from build123d import *

# Parameters (mm, degrees)
EXTRUDE_1_DEPTH = 2
SKETCH_4_R      = 5.25
SKETCH_4_R_2    = 3.25
EXTRUDE_4_DEPTH = 42.99


with BuildPart() as part:
    # Эскиз1 → Бобышка-Вытянуть1 (new body)
    with BuildSketch(Plane(origin=(0, 0, 0), x_dir=(1, 0, 0), z_dir=(0, 1, 0))):
        with BuildLine():
            Line((-21.495, 0), (21.495, 0))
            Line((21.495, 0), (21.495, -55.974685573))
            ThreePointArc((21.495, -55.974685573), (11.495, -64.530824352), (17.994657773, -75.974685573))
            Line((17.994657773, -75.974685573), (12.58, -130))
            Line((12.58, -130), (-12.58, -130))
            Line((-12.58, -130), (-17.994657773, -75.974685573))
            ThreePointArc((-17.994657773, -75.974685573), (-11.495, -64.530824352), (-21.495, -55.974685573))
            Line((-21.495, -55.974685573), (-21.495, 0))
        make_face()
    extrude(amount=EXTRUDE_1_DEPTH)

    # Эскиз4 → Бобышка-Вытянуть4 (add)
    with BuildSketch(Plane(origin=(21.495, 0, 0.569378428), x_dir=(0, 0, -1), z_dir=(1, 0, 0))):
        with Locations((0.569378428, 5.25)):
            Circle(SKETCH_4_R)
        with Locations((0.569378428, 5.25)):
            Circle(SKETCH_4_R_2, mode=Mode.SUBTRACT)
    extrude(amount=-EXTRUDE_4_DEPTH)


solid = part.part
Read the model definition and answer for the solid it produces. Units are mm, in the model's axes. Coordinates: 2 decimals unless noted, no trailing zeros. Order: outer loops, then holes, each group sorted by start corner. A loop starts at its lowest first (then second) coordinate and runs counter-clockwise, first axis right, second up. Notation, with made-up numbers: M 19,31 L 61,31 A14 cw 61,52 Z; hole C -35,77.25 d2. An arc over 180 degrees is marked long. Put each result on its own line as item: value. Start each with the question number.
Item 1: Consider probe 1 along Z at (x, y) = (7, 5.25); probe 2 along Y at (x, z) = (-6, 0); probe 3 along Y at (x, z) = (-16, 41.5). Determine where each line is inside the solid, lowest interval first. Write a range as [from, to].
Item 2: The mould has two halves that part along Z. Classify faces 1 (the face through (-15.25, 0.99, 103.37)), 2 (the face through (-11.462, 0.986, 64.728)), 3 (the face through (0, 2, 66)): +Z half, -Z half, draft (parallel to the pull), parting line (faces both ways), or undercut.
Item 3: Section B-B, the plane y = 5.25 is taken. Determine the outline of the cut face in (x, z) (3 decimals).
Item 4: Section D-D, the plane z = 44.5 is taken. Determine the outline of the cut face in (x, y) (3 decimals).
Item 5: Section C-C, the plane x = 10 is taken. Determine the outline of the cut face in (y, z).
Item 6: Section A-A, the plane x = -15.5 is taken. Determine the outline of the cut face in (y, z), plus the area to 3 significant figures.
Item 7: Given pin 1 Ø8 at (x, z) = (-1, 11) entering from +Y; pin 2 Ø3 at (x, y) = (0, 7.5) entering from +Z; pin 3 Ø2 at (x, y) = (4, 1) entering from -Z, each flat-ended and moving along its own axis, determine where each tip first touches the part or whether it passes through.
Computed:
1. probe 1: z = [-5.25, -3.25], [3.25, 5.25]
1. probe 2: y = [0, 2], [8.5, 10.5]
1. probe 3: y = [0, 2]
2. face 1: +Z half
2. face 2: undercut
2. face 3: draft
3. outline: M -21.495,-5.25 L 21.495,-5.25 L 21.495,-3.25 L -21.495,-3.25 Z; M -21.495,3.25 L 21.495,3.25 L 21.495,5.25 L -21.495,5.25 Z
4. outline: M -21.495,0 L 21.495,0 L 21.495,2 L -21.495,2 Z
5. outline: M 0,0 A5.25 ccw long 2,4.12 L 2,130 L 0,130 Z; hole C 5.25,0 d6.5
6. outline: M 0,0 A5.25 ccw long 2,4.12 L 2,58.02 L 0,58.02 Z; M 0,74.6 L 2,74.6 L 2,100.87 L 0,100.87 Z; hole C 5.25,0 d6.5
6. area: 216 mm2
7. pin 1: stops at y = 2
7. pin 2: stops at z = 5.2
7. pin 3: stops at z = -4.12
